from build123d import *

# Parameters (mm, degrees)
F0_W      = 150
F0_H      = 140
F1_DEPTH  = 2
F2_R      = 2.5
F3_DEPTH  = 2.001
F4_R      = 50
F4_R_2    = 49.75
F5_DEPTH  = 1
F7_DEPTH  = 2
F8_DEPTH  = 25
F9_DEPTH  = 2.001
F10_DEPTH = 25


# Not quite as in the source:
# - a feature names something its author has since deleted; it is built from what else it names


with BuildPart() as f1:
    # F0 (on Top) → F1 (new body)
    with BuildSketch(Plane.XY):
        Rectangle(F0_W, F0_H)
    extrude(amount=F1_DEPTH)

    # F2 (on face) → F3 (cut, through all)
    with BuildSketch(Plane.XY.offset(2)):
        Polygon((-75, 70), (-75, 41.5), (-46.5, 70), align=None)
        with Locations((-64, 57.6)):
            Circle(F2_R, mode=Mode.SUBTRACT)
        Polygon((-46.5, -70), (-75, -41.5), (-75, -70), align=None)
        with Locations((-64, -57.6)):
            Circle(F2_R, mode=Mode.SUBTRACT)
        with BuildLine():
            Line((-67.1845650673, -7), (-67.1845650673, 7))
            ThreePointArc((-67.1845650673, 7), (-67.9167981143, 8.767766953), (-69.6845650673, 9.5))
            Line((-69.6845650673, 9.5), (-75, 9.5))
            Line((-75, 9.5), (-75, -9.5))
            Line((-75, -9.5), (-69.6845650673, -9.5))
            ThreePointArc((-69.6845650673, -9.5), (-67.9167981143, -8.767766953), (-67.1845650673, -7))
        make_face()
        with BuildLine():
            Line((-26.5348799016, -66.5942596452), (-27.945, -70))
            Line((-27.945, -70), (-15, -70))
            Line((-15, -70), (-16.5005719841, -66.5208040123))
            ThreePointArc((-16.5005719841, -66.5208040123), (-21.5420765789, -63.2311459437), (-26.5348799016, -66.5942596452))
        make_face()
        with BuildLine():
            Line((-15, 70), (-27.945, 70))
            Line((-27.945, 70), (-26.6428877925, 66.4417666182))
            ThreePointArc((-26.6428877925, 66.4417666182), (-21.596779976, 63.2315774362), (-16.6462859149, 66.5873377421))
            Line((-16.6462859149, 66.5873377421), (-15, 70))
        make_face()
        with Locations((-64, 57.6)):
            Circle(F2_R)
        with Locations((-64, -57.6)):
            Circle(F2_R)
    extrude(amount=-F3_DEPTH, mode=Mode.SUBTRACT)

    # F4 (on face) → F5 (join)
    with BuildSketch(Plane.XY.offset(2)):
        with Locations((-3.16328, 0)):
            Circle(F4_R)
        with Locations((-3.16328, 0)):
            Circle(F4_R_2, mode=Mode.SUBTRACT)
    extrude(amount=F5_DEPTH)

    # F6 (on face) → F7 (join)
    with BuildSketch(Plane.XY.offset(2)):
        with BuildLine():
            Line((-3.16328, 49.75), (-3.16328, 7.5))
            Line((-3.16328, 7.5), (-2.66328, 7.5))
            Line((-2.66328, 7.5), (-0.16328, 49.6594653616))
            ThreePointArc((-0.16328, 49.6594653616), (-1.662597112, 49.7273611895), (-3.16328, 49.75))
        make_face()
        with BuildLine():
            Line((46.58672, 0), (4.33672, 0))
            Line((4.33672, 0), (4.33672, -0.5))
            Line((4.33672, -0.5), (46.4961853616, -3))
            ThreePointArc((46.4961853616, -3), (46.5640811895, -1.500682888), (46.58672, 0))
        make_face()
        with BuildLine():
            ThreePointArc((-52.8227453616, 3), (-52.8906411895, 1.500682888), (-52.91328, 0))
            Line((-52.91328, 0), (-10.66328, 0))
            Line((-10.66328, 0), (-10.66328, 0.5))
            Line((-10.66328, 0.5), (-52.8227453616, 3))
        make_face()
        with BuildLine():
            Line((-3.66328, -7.5), (-6.16328, -49.6594653616))
            ThreePointArc((-6.16328, -49.6594653616), (-4.663962888, -49.7273611895), (-3.16328, -49.75))
            Line((-3.16328, -49.75), (-3.16328, -7.5))
            Line((-3.16328, -7.5), (-3.66328, -7.5))
        make_face()
        with BuildLine():
            Line((4.33672, 0.5), (4.33672, 0))
            Line((4.33672, 0), (46.58672, 0))
            ThreePointArc((46.58672, 0), (46.5640811895, 1.500682888), (46.4961853616, 3))
            Line((46.4961853616, 3), (4.33672, 0.5))
        make_face()
        with BuildLine():
            Line((-10.66328, 0), (-52.91328, 0))
            ThreePointArc((-52.91328, 0), (-52.8906411895, -1.500682888), (-52.8227453616, -3))
            Line((-52.8227453616, -3), (-10.66328, -0.5))
            Line((-10.66328, -0.5), (-10.66328, 0))
        make_face()
        with BuildLine():
            Line((-2.66328, -7.5), (-3.16328, -7.5))
            Line((-3.16328, -7.5), (-3.16328, -49.75))
            ThreePointArc((-3.16328, -49.75), (-1.662597112, -49.7273611895), (-0.16328, -49.6594653616))
            Line((-0.16328, -49.6594653616), (-2.66328, -7.5))
        make_face()
        with BuildLine():
            ThreePointArc((-3.16328, 49.75), (-4.663962888, 49.7273611895), (-6.16328, 49.6594653616))
            Line((-6.16328, 49.6594653616), (-3.66328, 7.5))
            Line((-3.66328, 7.5), (-3.16328, 7.5))
            Line((-3.16328, 7.5), (-3.16328, 49.75))
        make_face()
    extrude(amount=F7_DEPTH)

    # F2 (on face) → F8 (cut)
    with BuildSketch(Plane.XY.offset(2)):
        with Locations((-64, 57.6)):
            Circle(F2_R)
        with Locations((-64, -57.6)):
            Circle(F2_R)
        with BuildLine():
            Line((-15, 70), (-27.945, 70))
            Line((-27.945, 70), (-26.6428877925, 66.4417666182))
            ThreePointArc((-26.6428877925, 66.4417666182), (-21.596779976, 63.2315774362), (-16.6462859149, 66.5873377421))
            Line((-16.6462859149, 66.5873377421), (-15, 70))
        make_face()
        with BuildLine():
            Line((-26.5348799016, -66.5942596452), (-27.945, -70))
            Line((-27.945, -70), (-15, -70))
            Line((-15, -70), (-16.5005719841, -66.5208040123))
            ThreePointArc((-16.5005719841, -66.5208040123), (-21.5420765789, -63.2311459437), (-26.5348799016, -66.5942596452))
        make_face()
    extrude(amount=-F8_DEPTH, mode=Mode.SUBTRACT)

    # F2 (on face) + F4 (on face) → F9 (cut, through all)
    with BuildSketch(Plane.XY.offset(2)):
        with Locations((-64, 57.6)):
            Circle(F2_R)
        with Locations((-64, -57.6)):
            Circle(F2_R)
        with BuildLine():
            Line((-15, 70), (-27.945, 70))
            Line((-27.945, 70), (-26.6428877925, 66.4417666182))
            ThreePointArc((-26.6428877925, 66.4417666182), (-21.596779976, 63.2315774362), (-16.6462859149, 66.5873377421))
            Line((-16.6462859149, 66.5873377421), (-15, 70))
        make_face()
    with BuildSketch(Plane.XY.offset(2)):
        with BuildLine():
            Line((-16.5005719841, -66.5208040123), (-15, -70))
            Line((-15, -70), (75, -70))
            Line((75, -70), (75, 70))
            Line((75, 70), (-15, 70))
            Line((-15, 70), (-16.6462859149, 66.5873377421))
            ThreePointArc((-16.6462859149, 66.5873377421), (-21.596779976, 63.2315774362), (-26.6428877925, 66.4417666182))
            Line((-26.6428877925, 66.4417666182), (-27.945, 70))
            Line((-27.945, 70), (-46.5, 70))
            Line((-46.5, 70), (-75, 41.5))
            Line((-75, 41.5), (-75, 9.5))
            Line((-75, 9.5), (-69.6845650673, 9.5))
            ThreePointArc((-69.6845650673, 9.5), (-67.9167981143, 8.767766953), (-67.1845650673, 7))
            Line((-67.1845650673, 7), (-67.1845650673, -7))
            ThreePointArc((-67.1845650673, -7), (-67.9167981143, -8.767766953), (-69.6845650673, -9.5))
            Line((-69.6845650673, -9.5), (-75, -9.5))
            Line((-75, -9.5), (-75, -41.5))
            Line((-75, -41.5), (-46.5, -70))
            Line((-46.5, -70), (-27.945, -70))
            Line((-27.945, -70), (-26.5348799016, -66.5942596452))
            ThreePointArc((-26.5348799016, -66.5942596452), (-21.5420765789, -63.2311459437), (-16.5005719841, -66.5208040123))
        make_face()
        with Locations((-3.16328, 0)):
            Circle(F4_R, mode=Mode.SUBTRACT)
    extrude(amount=-F9_DEPTH, mode=Mode.SUBTRACT)

    # F2 (on face) + F0 (on Top) → F10 (cut)
    with BuildSketch(Plane.XY.offset(2)):
        Polygon((-46.5, -70), (-75, -41.5), (-75, -70), align=None)
        with Locations((-64, -57.6)):
            Circle(F2_R, mode=Mode.SUBTRACT)
        Polygon((-75, 70), (-75, 41.5), (-46.5, 70), align=None)
        with Locations((-64, 57.6)):
            Circle(F2_R, mode=Mode.SUBTRACT)
        with BuildLine():
            Line((-67.1845650673, -7), (-67.1845650673, 7))
            ThreePointArc((-67.1845650673, 7), (-67.9167981143, 8.767766953), (-69.6845650673, 9.5))
            Line((-69.6845650673, 9.5), (-75, 9.5))
            Line((-75, 9.5), (-75, -9.5))
            Line((-75, -9.5), (-69.6845650673, -9.5))
            ThreePointArc((-69.6845650673, -9.5), (-67.9167981143, -8.767766953), (-67.1845650673, -7))
        make_face()
        with BuildLine():
            Line((-26.5348799016, -66.5942596452), (-27.945, -70))
            Line((-27.945, -70), (-15, -70))
            Line((-15, -70), (-16.5005719841, -66.5208040123))
            ThreePointArc((-16.5005719841, -66.5208040123), (-21.5420765789, -63.2311459437), (-26.5348799016, -66.5942596452))
        make_face()
        with BuildLine():
            Line((-15, 70), (-27.945, 70))
            Line((-27.945, 70), (-26.6428877925, 66.4417666182))
            ThreePointArc((-26.6428877925, 66.4417666182), (-21.596779976, 63.2315774362), (-16.6462859149, 66.5873377421))
            Line((-16.6462859149, 66.5873377421), (-15, 70))
        make_face()
    with BuildSketch(Plane.XY):
        Rectangle(F0_W, F0_H)
    extrude(amount=-F10_DEPTH, mode=Mode.SUBTRACT)


solid = f1.part
Can you work these out from the model? Positions are in its coordinate system, mm. A direction names the side the tool comes from. Give positions to 0.01 mm unless a question says otherwise; leave off trailing zeros. Write each loop counter-clockwise with the first axis right and the second up, starting at its lowest first coordinate (ties: lowest second). Pieces come first, ordered by that corner, then holes. Notation, with made-up numbers: (62, -35.5) -> (100, -35.5) arc R20 ccw to (100, -5.5) -> close; hole circle Ø11 at (24.25, 49). An arc over 180 degrees is marked (long way). Answer as a JSON object with one key per item and string values. Group by question number.
Item 1: I'm going to push flat-ended pins straight in: P1, Ø4, axis at x = -10.5, y = 31.5, coming from the -Z side; P2, Ø0.5, axis at y = 0, z = 3.5, coming from the +X side; P3, Ø4, axis at x = -28, y = -34, coming from the +Z side; P4, Ø2, axis at y = -19.5, z = 3, coming from the +X side. Where does each tip first touch, or does it pass through?
Item 2: Suppose I cut it at A-A (x = 24). Please give me the cut outline in (y, z).
Item 3: Please list where these lines run through material, in increasing order: line 1 (X direction, y = 13, z = 2.75); line 2 (Y direction, x = 16.5, z = 2.95); line 3 (Z direction, x = -28, y = 7.5). Write a range as [from, to].
Item 4: Suppose I cut it at C-C (z = 0.75). Please give me the cut outline in (x, y), plus the area to 3 significant figures.
Item 5: Suppose I cut it at D-D (y = -6). Please give me the cut outline in (x, z), plus the area to 3 significant figures.
Item 6: Suppose I cut it at B-B (y = 41.5). Please give me the cut outline in (x, z), plus the area to 3 significant figures.
Item 7: We'd pull the mould along Y, two halves only. Please class faces 1 (the face through (-3, -33, 4)), 2 (the face through (44.528, 15.019, 1.479)), 3 (the face through (25.712, 1.767, 2.986)): +Y half, -Y half, draft (parallel to the pull), parting line (faces both ways), or undercut.
Item 8: For faces 4 (the face through (-4, 1, 0)), 5 (the face through (-1.43, 28.28, 2.99)), which set-ups out of +Z, -Z, +X, -X, +Y, -Y let a thin tool reach every point of the face, with its end or its side?
Findings:
{
 "1": {"P1": "stops at z = 0", "P2": "stops at x = 46.59", "P3": "stops at z = 2", "P4": "stops at x = 43.29"},
 "2": {"outline": "(-41.98, 0) -> (41.98, 0) -> (41.98, 3) -> (41.68, 3) -> (41.68, 2) -> (1.67, 2) -> (1.67, 4) -> (-1.67, 4) -> (-1.67, 2) -> (-41.68, 2) -> (-41.68, 3) -> (-41.98, 3) -> close"},
 "3": {"line 1": "x = [-51.44, -51.18], [-3.99, -2.34], [44.86, 45.12]", "line 2": "y = [-45.97, -45.7], [-1.22, 1.22], [45.7, 45.97]", "line 3": "z = [0, 2]"},
 "4": {"outline": "circle Ø100 at (-3.16, 0)", "area": "7,850 mm²"},
 "5": {"outline": "(-52.8, 0) -> (46.48, 0) -> (46.48, 3) -> (46.22, 3) -> (46.22, 2) -> (-52.55, 2) -> (-52.55, 3) -> (-52.8, 3) -> close", "area": "199 mm²"},
 "6": {"outline": "(-31.05, 0) -> (24.72, 0) -> (24.72, 3) -> (24.27, 3) -> (24.27, 2) -> (-0.65, 2) -> (-0.65, 4) -> (-5.68, 4) -> (-5.68, 2) -> (-30.6, 2) -> (-30.6, 3) -> (-31.05, 3) -> close", "area": "123 mm²"},
 "7": {"face 1": "draft", "face 2": "parting line", "face 3": "undercut"},
 "8": {"face 4": "-Z, +X, -X, +Y, -Y", "face 5": "+Z"}
}
